Input: part model. Units: mm. Frame: model coordinates. A direction names the side the tool comes from. Give positions to 0.01 mm unless a question says otherwise; leave off trailing zeros. Order: outer loops, then holes, each group sorted by start corner. A loop starts at its lowest first (then second) coordinate and runs counter-clockwise, first axis right, second up. Notation, with made-up numbers: (20.5, 87.25) - (50.5, 87.25) arc R16 cw to (50.5, 117.25) - close; hole circle Ø9 at (81.25, 36). An arc over 180 degrees is marked (long way). Answer in a Markdown table with one row per item. Add a question column.
1. Section query A-A on z = 10.25. Return loops of the section in (x, y), and give its area (3 significant figures).
2. Ray query, line 1 (Z direction, x = 1, y = 0); line 2 (X direction, y = -0.45, z = 8.75); line 3 (Y direction, x = 0.1, z = 7.75). Return the intervals inside material, ascending. Write a range as [from, to].
3. Section query C-C on z = 7. Return loops of the section in (x, y), and give its area (3 significant figures).
4. Section query D-D on x = -2.05. Return loops of the section in (y, z).
5. Mould query, pull axis X, two halves, no side actions, for faces 3 (the face through (0, 0, 10.9)), 4 (the face through (0, 0, 0)), 5 (the face through (-1.5, 0.07, 4.93)). Classes: released by +X, released by -X, zero draft, split by the parting line, or undercut.
6. Section query B-B on x = 1.7. Return loops of the section in (y, z), and give its area (3 significant figures).
7. Contact query for flat-ended pins moving along their axis: pin 1 (1.5 mm diameter, centred on y = -2, z = 2.5, fed in from -X); pin 2 (1.5 mm diameter, centred on x = -2, y = 1, fed in from +Z); pin 3 (1 mm diameter, centred on y = -1.5, z = 5, fed in from -X). Output: stop coordinate, or through.
8. Access query for faces 1 (the face through (-0.607, -2.733, 10.782)), 2 (the face through (-1.2, -1.2, 10)). Directions: +Z, -Z, +X, -X, +Y, -Y. A direction counts if a zero-diameter tool reaches every point of the face in a straight line with its end or side. Return the directions, or none.
```python
from build123d import *

# Parameters (mm, degrees)
SKETCH1_R          = 1.5
BASE_EXTRUDE_DEPTH = 10
CUT_EXTRUDE1_DEPTH = 1.799999969
CUT_EXTRUDE1_TAPER = 2


with BuildPart() as part:
    # Sketch1 → Base-Extrude (new body)
    with BuildSketch(Plane.XY):
        Circle(SKETCH1_R)
    extrude(amount=BASE_EXTRUDE_DEPTH)

    # Sketch6 → Boss-Revolve2 (revolve)
    with BuildSketch(Plane(origin=(0, 0, 0), x_dir=(1, 0, 0), z_dir=(0, 1, 0))):
        with BuildLine():
            Line((0, -10), (2.7999999, -10))
            Line((2.7999999, -10), (2.7999999, -11.54246308))
            ThreePointArc((2.7999999, -11.54246308), (1.46418655, -12.180811406), (0, -12.4))
            Line((0, -12.4), (0, -10))
        make_face()
    revolve(axis=Axis((0, 0, -0.393620135), (0, 0, 1)))

    # Sketch7 → Cut-Extrude1 (cut)
    with BuildSketch(Plane(origin=(0, 0, 12.7000001), x_dir=(-1, 0, 0), z_dir=(0, 0, -1))):
        with BuildLine():
            ThreePointArc((0.205000004, 1.48592565), (0, 1.500000013), (-0.205000004, 1.48592565))
            Line((-0.205000004, 1.48592565), (-0.205000004, 0.708178558))
            ThreePointArc((-0.205000004, 0.708178558), (-0.35072876, 0.355344481), (-0.702967546, 0.208182689))
            Line((-0.702967546, 0.208182689), (-1.48592565, 0.205000004))
            ThreePointArc((-1.48592565, 0.205000004), (-1.500000013, 0), (-1.48592565, -0.205000004))
            Line((-1.48592565, -0.205000004), (-0.702967546, -0.208182689))
            ThreePointArc((-0.702967546, -0.208182689), (-0.35072876, -0.355344481), (-0.205000004, -0.708178558))
            Line((-0.205000004, -0.708178558), (-0.205000004, -1.48592565))
            ThreePointArc((-0.205000004, -1.48592565), (0, -1.500000013), (0.205000004, -1.48592565))
            Line((0.205000004, -1.48592565), (0.205000004, -0.708178558))
            ThreePointArc((0.205000004, -0.708178558), (0.35072876, -0.355344481), (0.702967546, -0.208182689))
            Line((0.702967546, -0.208182689), (1.48592565, -0.205000004))
            ThreePointArc((1.48592565, -0.205000004), (1.500000013, 0), (1.48592565, 0.205000004))
            Line((1.48592565, 0.205000004), (0.702967546, 0.208182689))
            ThreePointArc((0.702967546, 0.208182689), (0.35072876, 0.355344481), (0.205000004, 0.708178558))
            Line((0.205000004, 0.708178558), (0.205000004, 1.48592565))
        make_face()
    extrude(amount=CUT_EXTRUDE1_DEPTH, taper=CUT_EXTRUDE1_TAPER, mode=Mode.SUBTRACT)


solid = part.part
```
Answer:
| question | item | result |
|---|---|---|
| 1 | outline | circle Ø5.6 at (0, 0) |
| 1 | area | 24.6 mm² |
| 2 | line 1 | z = [0, 10.9] |
| 2 | line 2 | x = [-1.43, 1.43] |
| 2 | line 3 | y = [-1.5, 1.5] |
| 3 | outline | circle Ø3 at (0, 0) |
| 3 | area | 7.07 mm² |
| 4 | outline | (-1.91, 10) - (1.91, 10) - (1.91, 11.54) arc R4.56 ccw to (-1.91, 11.54) - close |
| 5 | face 3 | undercut |
| 5 | face 4 | zero draft |
| 5 | face 5 | split by the parting line |
| 6 | outline | (-2.22, 10) - (2.22, 10) - (2.22, 11.54) arc R4.7 ccw to (-2.22, 11.54) - close |
| 6 | area | 8.54 mm² |
| 7 | pin 1 | stops at x = -0.83 |
| 7 | pin 2 | stops at z = 12.17 |
| 7 | pin 3 | stops at x = -1.12 |
| 8 | face 1 | +Z, -Z |
| 8 | face 2 | -Z |
